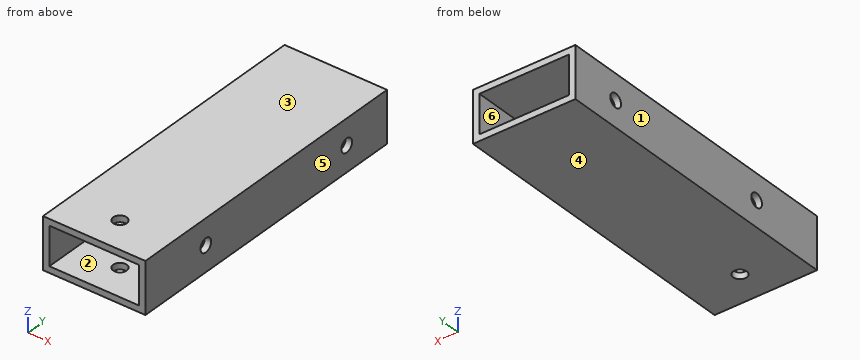
from build123d import *

# Parameters (mm, degrees)
SKETCH1_W           = 50.8
SKETCH1_H           = 25.4
SKETCH1_W_2         = 44.45
SKETCH1_H_2         = 19.05
BOSS_EXTRUDE1_DEPTH = 152.4
SKETCH2_R           = 3.3782
CUT_EXTRUDE1_DEPTH  = 51.8
SKETCH3_R           = 3.3782
CUT_EXTRUDE2_DEPTH  = 26.4


with BuildPart() as part:
    # Sketch1 → Boss-Extrude1 (new body)
    with BuildSketch(Plane(origin=(0, 0, 0), x_dir=(1, 0, 0), z_dir=(0, 1, 0))):
        with Locations((25.4, 12.7)):
            Rectangle(SKETCH1_W, SKETCH1_H)
        with Locations((25.4, 12.7)):
            Rectangle(SKETCH1_W_2, SKETCH1_H_2, mode=Mode.SUBTRACT)
    extrude(amount=BOSS_EXTRUDE1_DEPTH)

    # Sketch2 → Cut-Extrude1 (cut, through all)
    with BuildSketch(Plane.ZY):
        with Locations((-12.7, 127)):
            Circle(SKETCH2_R)
        with Locations((-12.7, 38.1)):
            Circle(SKETCH2_R)
    extrude(amount=-CUT_EXTRUDE1_DEPTH, mode=Mode.SUBTRACT)

    # Sketch3 → Cut-Extrude2 (cut, through all)
    with BuildSketch(Plane(origin=(0, 0, -25.4), x_dir=(-1, 0, 0), z_dir=(0, 0, -1))):
        with Locations((-25.4, 16.2687)):
            Circle(SKETCH3_R)
    extrude(amount=-CUT_EXTRUDE2_DEPTH, mode=Mode.SUBTRACT)


solid = part.part
Build history of the part. All positions in model axes, mm. Face numbers are marked on the shaded views. A direction names the side the tool comes from. Give positions to 0.01 mm unless a question says otherwise; leave off trailing zeros. Loops run counter-clockwise (first coordinate to the right, second up) from the corner with the lowest first, then second, coordinate; pieces in that order, holes last. Notation, with made-up numbers: (77.5, -4) - (111.5, -4) arc R5 cw to (111.5, 2) - close; hole circle Ø3 at (44, 44). An arc over 180 degrees is marked (long way). Write item = value, one per line. Start each with the question number.
1) Probe probe 1 along Y at (x, z) = (0.8, -12.7); probe 2 along Z at (x, y) = (31, 27) (3 decimals); probe 3 along X at (y, z) = (18.5, -22) (3 decimals). List the from-to ranges inside material, lowest first. Write a range as from..to.
2) Band-saw the part on A-A on y = 113. Give the cut face in (x, z) (3 decimals).
3) Band-saw the part on C-C on z = -12.7. Give the cut face in (x, y) (3 decimals), plus the area to 3 significant figures.
4) Band-saw the part on D-D on x = 44.5. Give the cut face in (y, z) (3 decimals).
5) Band-saw the part on B-B on x = 25.4. Give the cut face in (y, z) (1 decimal), plus the area to 3 significant figures.
6) Pull direction Z, two halves, no side cores. Call the marked faces 3, 4, 5 and 6: +Z half, -Z half, draft (parallel to the pull), parting line (faces both ways), or undercut.
7) Tool access for the marked faces 1 and 2: list every direction of +Z, -Z, +X, -X, +Y, -Y with a clear straight run to the whole face (end or side of a thin tool).
Final values:
q1.probe_1 = 0..34.72, 41.48..123.62, 130.38..152.4
q1.probe_2 = -25.4..-22.225, -3.175..0
q1.probe_3 = 0..3.175, 47.625..50.8
q2.outline = (0, -25.4) - (50.8, -25.4) - (50.8, 0) - (0, 0) - close; hole (3.175, -22.225) - (47.625, -22.225) - (47.625, -3.175) - (3.175, -3.175) - close
q3.outline = (0, 0) - (3.175, 0) - (3.175, 34.722) - (0, 34.722) - close; (0, 41.478) - (3.175, 41.478) - (3.175, 123.622) - (0, 123.622) - close; (0, 130.378) - (3.175, 130.378) - (3.175, 152.4) - (0, 152.4) - close; (47.625, 0) - (50.8, 0) - (50.8, 34.722) - (47.625, 34.722) - close; (47.625, 41.478) - (50.8, 41.478) - (50.8, 123.622) - (47.625, 123.622) - close; (47.625, 130.378) - (50.8, 130.378) - (50.8, 152.4) - (47.625, 152.4) - close
q3.area = 882 mm²
q4.outline = (0, -25.4) - (152.4, -25.4) - (152.4, -22.225) - (0, -22.225) - close; (0, -3.175) - (152.4, -3.175) - (152.4, 0) - (0, 0) - close
q5.outline = (0, -25.4) - (12.9, -25.4) - (12.9, -22.2) - (0, -22.2) - close; (0, -3.2) - (12.9, -3.2) - (12.9, 0) - (0, 0) - close; (19.6, -25.4) - (152.4, -25.4) - (152.4, -22.2) - (19.6, -22.2) - close; (19.6, -3.2) - (152.4, -3.2) - (152.4, 0) - (19.6, 0) - close
q5.area = 925 mm²
q6.face_3 = +Z half
q6.face_4 = -Z half
q6.face_5 = draft
q6.face_6 = undercut
q7.face_1 = +Z, -Z, -X, +Y, -Y
q7.face_2 = +Y, -Y
